Verification items for this drawing (mm, ordinates from the low corner). Coordinates: 2 decimals unless noted, no trailing zeros. Write each loop counter-clockwise with the first axis right and the second up, starting at its lowest first coordinate (ties: lowest second). Pieces come first, ordered by that corner, then holes. Notation, with made-up numbers: M -9.5,55 L 6.5,55 A19 cw 6.5,89 Z; hole C -11.5,-31 d10. An arc over 180 degrees is marked long. Put each result on its own line as item: value. Start each with the question number.
1) Cross-section at B-B on x = 40. Record the cut outline in (y, z), plus the area to 3 significant figures.
2) Cross-section at A-A on z = 40. Record the cut outline in (x, y).
3) Scan lines: line 1 along Z through (x, y) = (40, 4.75); line 2 along Z through (x, y) = (39, 9.25); line 3 along X through (y, z) = (6.25, 19.5). Record each from-to range of solid material in increasing order.
4) Gauge pin test, flat ends, axial feed: pin 1 (1.5 mm diameter, centred on x = 8, y = 2, fed in from -Z); pin 2 (5 mm diameter, centred on y = 5.5, z = 65, fed in from +X); pin 3 (2 mm diameter, centred on y = 6, z = 50.5, fed in from +X). Record the tip position at first contact, or that the pin passes through.
5) Cross-section at C-C on z = 19. Record the cut outline in (x, y).
6) Mould release check, pull along Z, two halves, no side actions. Record for the marked faces 1, 2, 3 and 4: released by +Z, released by -Z, zero draft, split by the parting line, or undercut.
7) Cross-section at D-D on x = 27.5. Record the cut outline in (y, z), plus the area to 3 significant figures.
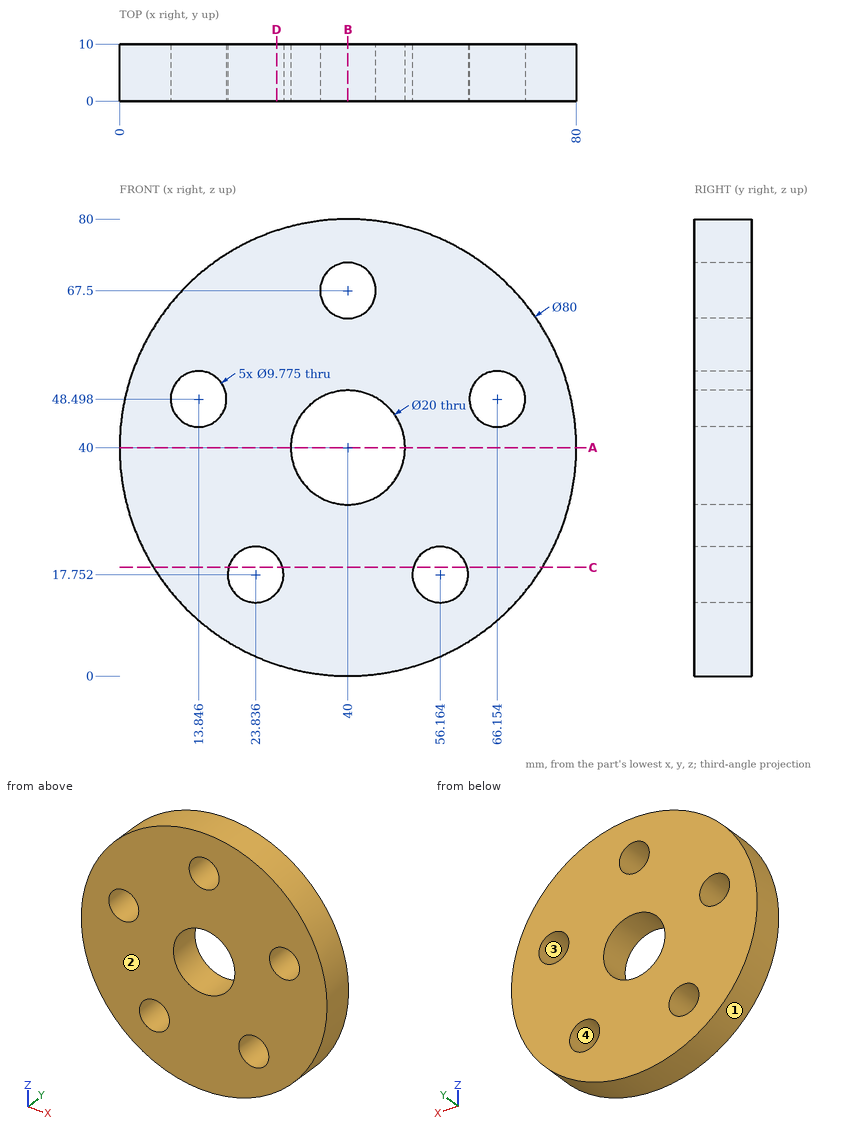
Answer key:
1. outline: M 0,0 L 10,0 L 10,30 L 0,30 Z; M 0,50 L 10,50 L 10,62.61 L 0,62.61 Z; M 0,72.39 L 10,72.39 L 10,80 L 0,80 Z
1. area: 502 mm²
2. outline: M 0,0 L 30,0 L 30,10 L 0,10 Z; M 50,0 L 80,0 L 80,10 L 50,10 Z
3. line 1: z = 0 to 30, 50 to 62.61, 72.39 to 80
3. line 2: z = 0.01 to 30.05, 49.95 to 62.72, 72.28 to 79.99
3. line 3: x = 5.65 to 19.27, 28.4 to 51.6, 60.73 to 74.35
4. pin 1: stops at z = 15.03
4. pin 2: stops at x = 73.07
4. pin 3: stops at x = 78.86
5. outline: M 5.96,0 L 19.11,0 L 19.11,10 L 5.96,10 Z; M 28.56,0 L 51.44,0 L 51.44,10 L 28.56,10 Z; M 60.89,0 L 74.04,0 L 74.04,10 L 60.89,10 Z
6. face 1: split by the parting line
6. face 2: zero draft
6. face 3: undercut
6. face 4: undercut
7. outline: M 0,2 L 10,2 L 10,14.52 L 0,14.52 Z; M 0,20.99 L 10,20.99 L 10,78 L 0,78 Z
7. area: 695 mm²
